from build123d import *

# Parameters (mm, degrees)
CROQUIS1_W               = 50
CROQUIS1_H               = 20
SALIENTE_EXTRUIR1_DEPTH  = 11
REDONDEO1_R              = 5
CROQUIS2_OUTSIDE_W       = 33.634
CROQUIS2_OUTSIDE_H       = 35.634
CORTAR_EXTRUIR1_DEPTH    = 14
CROQUIS3_R               = 1.5
CORTAR_EXTRUIR2_DEPTH    = 34.85262176
SALIENTE_EXTRUIR6_DEPTH  = 8
CROQUIS9_R               = 2.7
CORTAR_EXTRUIR5_DEPTH    = 41.124805295
SALIENTE_EXTRUIR7_DEPTH  = 6
SALIENTE_EXTRUIR7_DRAFT  = 7
REDONDEO2_R              = 1
CORTAR_EXTRUIR6_START    = -6
CORTAR_EXTRUIR6_DEPTH    = 6
CROQUIS15_W              = 2
CROQUIS15_H              = 5
SALIENTE_EXTRUIR10_DEPTH = 5.5
CROQUIS16_R              = 1.5
CORTAR_EXTRUIR7_DEPTH    = 42.988093643
CROQUIS17_R              = 1
SALIENTE_EXTRUIR11_DEPTH = 1.5
CORTAR_EXTRUIR8_START    = -5.5
CROQUIS18_W              = 2
CROQUIS18_H              = 5
CORTAR_EXTRUIR8_DEPTH    = 79.039644333


with BuildPart() as part:
    # Croquis1 → Saliente-Extruir1 (new, symmetric)
    with BuildSketch(Plane(origin=(0, 0, 0), x_dir=(1, 0, 0), z_dir=(0, 1, 0))):
        Rectangle(CROQUIS1_W, CROQUIS1_H)
    extrude(amount=SALIENTE_EXTRUIR1_DEPTH, both=True)

    # Redondeo1
    redondeo1_edges = [part.edges().sort_by_distance(p)[0] for p in [
        (-25, 11, 0),
        (-25, -11, 0),
    ]]
    fillet(redondeo1_edges, radius=REDONDEO1_R)

    # Croquis2 outside → Cortar-Extruir1 (cut)
    with BuildSketch(Plane(origin=(25, 0, 0), x_dir=(0, 0, -1), z_dir=(1, 0, 0))):
        Rectangle(CROQUIS2_OUTSIDE_W, CROQUIS2_OUTSIDE_H)
        with BuildLine():
            Line((-10, 7), (-10, -7))
            ThreePointArc((-10, -7), (-0.75, -11), (8.5, -7))
            Line((8.5, -7), (8.5, 7))
            ThreePointArc((8.5, 7), (-0.75, 11), (-10, 7))
        make_face(mode=Mode.SUBTRACT)
    extrude(amount=-CORTAR_EXTRUIR1_DEPTH, mode=Mode.SUBTRACT)

    # Croquis3 → Cortar-Extruir2 (cut, through all)
    with BuildSketch(Plane(origin=(0, 0, -10), x_dir=(-1, 0, 0), z_dir=(0, 0, -1))):
        with Locations((-6, 8)):
            Circle(CROQUIS3_R)
        with Locations(Location((-6, -8, 0), (0, 0, 180))):
            Circle(CROQUIS3_R)
    extrude(amount=-CORTAR_EXTRUIR2_DEPTH, mode=Mode.SUBTRACT)

    # Croquis8 → Saliente-Extruir6 (add)
    with BuildSketch(Plane(origin=(25, 0, 0), x_dir=(0, 0, -1), z_dir=(1, 0, 0))):
        with BuildLine():
            Line((-9, 6.594309595), (-9, -6.594309595))
            ThreePointArc((-9, -6.594309595), (-0.75, -10), (7.5, -6.594309595))
            Line((7.5, -6.594309595), (7.5, 6.594309595))
            ThreePointArc((7.5, 6.594309595), (-0.75, 10), (-9, 6.594309595))
        make_face()
    extrude(amount=SALIENTE_EXTRUIR6_DEPTH)

    # Croquis9 → Cortar-Extruir5 (cut, through all)
    with BuildSketch(Plane.XY.offset(10)):
        with Locations((-13, 0)):
            Circle(CROQUIS9_R)
    extrude(amount=-CORTAR_EXTRUIR5_DEPTH, mode=Mode.SUBTRACT)


with BuildPart() as saliente_extruir7_tool:
    # Croquis11 → Saliente-Extruir7 (with draft: the straight prism first)
    with BuildSketch(Plane(origin=(33, 0, 0), x_dir=(0, 0, -1), z_dir=(1, 0, 0))):
        with BuildLine():
            Line((-9, 6.594309595), (-9, -6.594309595))
            ThreePointArc((-9, -6.594309595), (-0.75, -10), (7.5, -6.594309595))
            Line((7.5, -6.594309595), (7.5, 6.594309595))
            ThreePointArc((7.5, 6.594309595), (-0.75, 10), (-9, 6.594309595))
        make_face()
    extrude(amount=SALIENTE_EXTRUIR7_DEPTH)
    # Saliente-Extruir7: the draft: its side faces are tilted about the plane it starts from
    saliente_extruir7_sides = [saliente_extruir7_tool.faces().sort_by_distance(p)[0] for p in [
        (36, 0, 9),
        (36, -10, 0.75),
        (36, 0, -7.5),
        (36, 10, 0.75),
    ]]
    draft(saliente_extruir7_sides, Plane(origin=(33, 0, 0), x_dir=(0, 0, -1), z_dir=(1, 0, 0)), SALIENTE_EXTRUIR7_DRAFT)


with BuildPart() as part_1:
    add(part.part)

    # Saliente-Extruir7: add saliente_extruir7_tool
    add(saliente_extruir7_tool.part)

    # Redondeo2
    redondeo2_edges = [part_1.edges().sort_by_distance(p)[0] for p in [
        (39, 0, -6.763292635),
        (39, -9.263292635, 0.75),
        (39, 0, 8.263292635),
        (39, 9.263292635, 0.75),
    ]]
    fillet(redondeo2_edges, radius=REDONDEO2_R - 0.0001)  # a hair under: the kernel refuses the full size

    # Croquis14 → Cortar-Extruir6 (cut)
    with BuildSketch(Plane(origin=(39, 0, 0), x_dir=(0, 0, -1), z_dir=(1, 0, 0)).offset(CORTAR_EXTRUIR6_START)):
        with BuildLine():
            Line((-2.25, 9.903408743), (-2.25, 8.403408743))
            ThreePointArc((-2.25, 8.403408743), (-0.75, 6.903408743), (0.75, 8.403408743))
            Line((0.75, 8.403408743), (0.75, 9.903408743))
            ThreePointArc((0.75, 9.903408743), (-0.75, 10), (-2.25, 9.903408743))
        make_face()
        with BuildLine():
            Line((-2.25, -9.903408743), (-2.25, -8.403408743))
            ThreePointArc((-2.25, -8.403408743), (-0.75, -6.903408743), (0.75, -8.403408743))
            Line((0.75, -8.403408743), (0.75, -9.903408743))
            ThreePointArc((0.75, -9.903408743), (-0.75, -10), (-2.25, -9.903408743))
        make_face()
    extrude(amount=CORTAR_EXTRUIR6_DEPTH, mode=Mode.SUBTRACT)

    # Croquis15 → Saliente-Extruir10 (add)
    with BuildSketch(Plane.ZY.offset(25)):
        Rectangle(CROQUIS15_W, CROQUIS15_H)
    extrude(amount=SALIENTE_EXTRUIR10_DEPTH)

    # Croquis16 → Cortar-Extruir7 (cut, through all)
    with BuildSketch(Plane.XY.offset(1)):
        with Locations((-27.75, 0)):
            Circle(CROQUIS16_R)
    extrude(amount=-CORTAR_EXTRUIR7_DEPTH, mode=Mode.SUBTRACT)

    # Croquis17 → Saliente-Extruir11 (add)
    with BuildSketch(Plane(origin=(39, 0, 0), x_dir=(0, 0, -1), z_dir=(1, 0, 0))):
        with Locations((-0.75, 0)):
            Circle(CROQUIS17_R)
    extrude(amount=SALIENTE_EXTRUIR11_DEPTH)

    # Croquis18 → Cortar-Extruir8 (cut, through all)
    with BuildSketch(Plane.ZY.offset(30.5).offset(CORTAR_EXTRUIR8_START)):
        Rectangle(CROQUIS18_W, CROQUIS18_H)
    extrude(amount=CORTAR_EXTRUIR8_DEPTH, mode=Mode.SUBTRACT)


solid = part_1.part
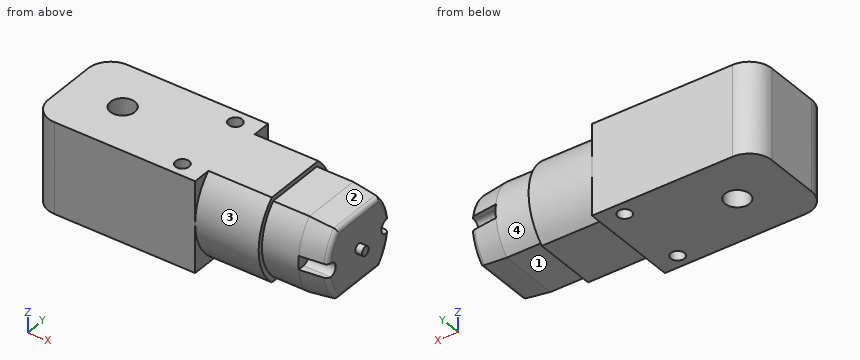
Read the model definition and answer for the solid it produces. Units are mm, in the model's axes. Face numbers are marked on the shaded views. A direction names the side the tool comes from. Coordinates: 2 decimals unless noted, no trailing zeros. Write each loop counter-clockwise with the first axis right and the second up, starting at its lowest first coordinate (ties: lowest second). Pieces come first, ordered by that corner, then holes. Notation, with made-up numbers: M -36,-22 L -27,-22 A8 cw -27,-9 Z; hole C 7,-28.75 d1. An arc over 180 degrees is marked long. Use a Markdown table: item, result.
Q1. Straight lines are drawn through the part: L1, parallel to Y at x = 6, z = 2; L2, parallel to Y at x = -13, z = -1; L3, parallel to Z at x = 34.5, y = -8.75. For each, find the intervals that lie inside material, in ascending order. Write a range as [from, to].
Answer block:
| item | result |
|---|---|
| L1 | y = [-11, -9.5], [-6.5, 6.5], [9.5, 11] |
| L2 | y = [-11, -2.7], [2.7, 11] |
| L3 | z = [-4.09, -0.75], [2.25, 5.59] |
Q2. The part is cut by section C-C, the plane y = 0. Write down the section's boundary in (x, z), then the cut area to 3 significant figures.
Answer block:
| item | result |
|---|---|
| outline | M -25,-10 L -15.7,-10 L -15.7,10 L -25,10 Z; M -10.3,-10 L 11,-10 L 11,-8.5 L 25,-8.5 L 25,-7.5 L 33,-7.5 L 38.12,-6.87 A1 ccw 39,-5.88 L 39,-0.25 L 40.5,-0.25 L 40.5,1.75 L 39,1.75 L 39,7.38 A1 ccw 38.12,8.37 L 33,9 L 25,9 L 25,10 L -10.3,10 Z |
| area | 1,100 mm2 |
Q3. The part is cut by section A-A, the plane x = 6. Write down the section's boundary in (y, z).
Answer block:
| item | result |
|---|---|
| outline | M -11,-10 L -9.5,-10 L -9.5,10 L -11,10 Z; M -6.5,-10 L 6.5,-10 L 6.5,10 L -6.5,10 Z; M 9.5,-10 L 11,-10 L 11,10 L 9.5,10 Z |
Q4. The part is cut by section D-D, the plane x = 26. Write down the section's boundary in (y, z), then the cut area to 3 significant figures.
Answer block:
| item | result |
|---|---|
| outline | M -6.59,-7.5 L 6.59,-7.5 A11.7 ccw 6.59,9 L -6.59,9 A11.7 ccw Z |
| area | 295 mm2 |
Q5. The part is cut by section B-B, the plane x = -13. Write down the section's boundary in (y, z).
Answer block:
| item | result |
|---|---|
| outline | M -11,-10 L -2.7,-10 L -2.7,10 L -11,10 Z; M 2.7,-10 L 11,-10 L 11,10 L 2.7,10 Z |
Q6. Which of the six approach directions +Z, -Z, +X, -X, +Y, -Y give full straight-line access (tool end or side, diameter ignored) to the marked faces 1, 2, 3 and 4?
Answer block:
| item | result |
|---|---|
| face 1 | -Z, +X, +Y, -Y |
| face 2 | +Z, +X, +Y, -Y |
| face 3 | +X, -Y |
| face 4 | +X, +Y |
Q7. Each of these flat-tipped pins is pushed along its axis until it touches: pin 1 Ø1.5 at (y, z) = (7.5, 1) entering from +X; pin 2 Ø2.5 at (x, y) = (31, 3) entering from -Z; pin 3 Ø6.5 at (x, y) = (31, 2.5) entering from +Z. Where does it stop, or does it pass through?
Answer block:
| item | result |
|---|---|
| pin 1 | stops at x = 39 |
| pin 2 | stops at z = -7.5 |
| pin 3 | stops at z = 9 |
